Work out the finished part from the listing and answer in its coordinate system (mm). Round coordinates to 2 decimals unless told otherwise and drop trailing zeros. Write each loop counter-clockwise with the first axis right and the second up, starting at its lowest first coordinate (ties: lowest second). Pieces come first, ordered by that corner, then holes. Notation, with made-up numbers: (-37.5, -2) -> (-7.5, -2) arc R14 ccw to (-7.5, 4) -> close; hole circle Ø5 at (49, -31). An arc over 180 degrees is marked (long way). One line per item, written item: value.
```python
from build123d import *

# Parameters (mm, degrees)
SKETCH1_R                  = 1.25
BOSS_EXTRUDE1_DEPTH        = 5
BOSS_EXTRUDE2_START        = -5
BOSS_EXTRUDE2_DEPTH        = 5
F_2_0_2_DIAMETER_HOLE2_D   = 2
FILLET2_R                  = 3
F_2_8_2_8_DIAMETER_HOLE1_D = 2.8


with BuildPart() as part:
    # Sketch1 → Boss-Extrude1 (new body)
    with BuildSketch(Plane(origin=(0, 0, 0), x_dir=(1, 0, 0), z_dir=(0, 1, 0))):
        with BuildLine():
            Line((29, 74), (-29, 74))
            ThreePointArc((-29, 74), (-45.770509831, 70.041019662), (-59, 59))
            Line((-59, 59), (-59, 0))
            Line((-59, 0), (-59, -15))
            ThreePointArc((-59, -15), (-67.992720962, -23.992720962), (-76.985441925, -15))
            Line((-76.985441925, -15), (-75, 0))
            Line((-75, 0), (-75, 60))
            ThreePointArc((-75, 60), (-56.459060435, 81.837226001), (-29, 90))
            Line((-29, 90), (29, 90))
            ThreePointArc((29, 90), (56.459060435, 81.837226001), (75, 60))
            Line((75, 60), (75, 0))
            Line((75, 0), (76.985441925, -15))
            ThreePointArc((76.985441925, -15), (67.992720962, -23.992720962), (59, -15))
            Line((59, -15), (59, 0))
            Line((59, 0), (59, 59))
            ThreePointArc((59, 59), (45.770509831, 70.041019662), (29, 74))
        make_face()
        with Locations(Location((67, 5, 0), (0, 0, 270))):
            Circle(SKETCH1_R, mode=Mode.SUBTRACT)
        with Locations(Location((68.915666574, -15, 0), (0, 0, 270))):
            Circle(SKETCH1_R, mode=Mode.SUBTRACT)
        with Locations(Location((-68.915666574, -15, 0), (0, 0, 90))):
            Circle(SKETCH1_R, mode=Mode.SUBTRACT)
        with Locations(Location((-67, 5, 0), (0, 0, 90))):
            Circle(SKETCH1_R, mode=Mode.SUBTRACT)
    extrude(amount=BOSS_EXTRUDE1_DEPTH)

    # Sketch2 → Boss-Extrude2 (add)
    with BuildSketch(Plane(origin=(0, 5, 0), x_dir=(1, 0, 0), z_dir=(0, 1, 0)).offset(BOSS_EXTRUDE2_START)):
        with BuildLine():
            Line((52, 45.986664295), (59, 39.986664295))
            Line((59, 39.986664295), (59, 51.986664295))
            ThreePointArc((59, 51.986664295), (54.390227771, 50.281398562), (52, 45.986664295))
        make_face()
        with BuildLine():
            ThreePointArc((26.500025406, 74), (29.864997094, 70.489268948), (33.490587946, 73.730157398))
            ThreePointArc((33.490587946, 73.730157398), (31.249344079, 73.932478561), (29, 74))
            Line((29, 74), (26.500025406, 74))
        make_face()
        with BuildLine():
            ThreePointArc((-33.490587946, 73.730157398), (-29.864997094, 70.489268948), (-26.500025406, 74))
            Line((-26.500025406, 74), (-29, 74))
            ThreePointArc((-29, 74), (-31.249344079, 73.932478561), (-33.490587946, 73.730157398))
        make_face()
        with BuildLine():
            Line((-6.92820323, 90), (6.92820323, 90))
            ThreePointArc((6.92820323, 90), (0, 94), (-6.92820323, 90))
        make_face()
        with BuildLine():
            ThreePointArc((-52, 45.986664295), (-54.390227771, 50.281398562), (-59, 51.986664295))
            Line((-59, 51.986664295), (-59, 39.986664295))
            Line((-59, 39.986664295), (-52, 45.986664295))
        make_face()
    extrude(amount=BOSS_EXTRUDE2_DEPTH)

    # Ø2.0 (2) Diameter Hole2 (through all)
    with Locations(Plane(origin=(0, 5, 0), x_dir=(1, 0, 0), z_dir=(0, 1, 0))):
        with Locations((30, 73.986664295), (56, 47.986664295), (-30, 73.986664295), (-56, 47.986664295)):
            Hole(F_2_0_2_DIAMETER_HOLE2_D / 2)

    # Fillet2
    fillet2_edges = [part.edges().sort_by_distance(p)[0] for p in [
        (52, 2.5, -45.986664295),
        (59, 2.5, -51.986664295),
        (59, 2.5, -39.986664295),
        (59, 2.5, -59),
        (-59, 2.5, -59),
        (-75, 2.5, -60),
        (75, 2.5, -60),
        (-6.92820323, 2.5, -90),
        (6.92820323, 2.5, -90),
        (-26.500025406, 2.5, -74),
        (-33.490587946, 2.5, -73.730157398),
        (-52, 2.5, -45.986664295),
        (-59, 2.5, -39.986664295),
        (-59, 2.5, -51.986664295),
        (26.500025406, 2.5, -74),
        (33.490587946, 2.5, -73.730157398),
    ]]
    fillet(fillet2_edges, radius=FILLET2_R)

    # Ø2.8 (2.8) Diameter Hole1 (through all)
    with Locations(Plane(origin=(0, 5, 0), x_dir=(1, 0, 0), z_dir=(0, 1, 0))):
        with Locations((0, 86)):
            Hole(F_2_8_2_8_DIAMETER_HOLE1_D / 2)


solid = part.part
```
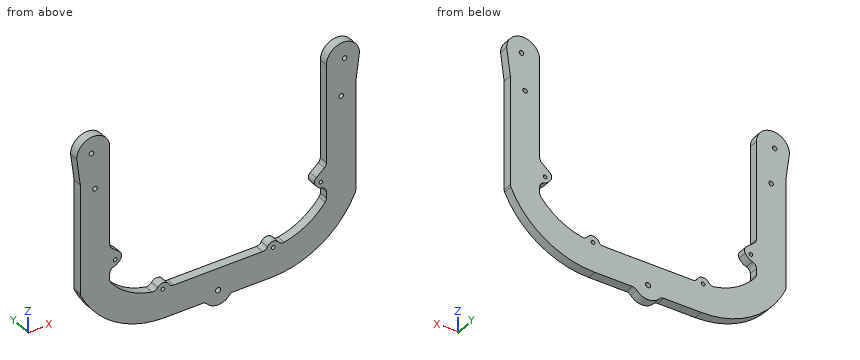
(1) Find section D-D on x = 40. Give the vertices of the cut face in (y, z).
Reported:
outline: (0, -88.78) -> (5, -88.78) -> (5, -72.35) -> (0, -72.35) -> close
(2) Flat-ended cylindrical pins translate along their axes: pin 1 Ø3 at (y, z) = (3.5, -57) entering from +X; pin 2 Ø3 at (x, y) = (-30.5, 1.5) entering from -Z; pin 3 Ø1 at (y, z) = (3.5, -61.5) entering from +X; pin 4 Ø1.5 at (x, z) = (67, -5) entering from +Y. Find the tip coordinate at first contact, or state that the pin passes through.
Reported:
pin 1: stops at x = 75
pin 2: stops at z = -90
pin 3: stops at x = 74.55
pin 4: passes through
(3) Consider probe 1 along X at (y, z) = (3.25, -32.5); probe 2 along Z at (x, y) = (30, 3); probe 3 along Z at (x, y) = (-56, 2.2). Determine where each line is inside the solid, lowest interval first.
Reported:
probe 1: x = -75 to -59, 59 to 75
probe 2: z = -89.99 to -74.99, -72.99 to -70.49
probe 3: z = -82.13 to -62.52, -51.32 to -48.99, -46.99 to -42.56
(4) Find section C-C on y = 3.75. Give the number of separate pieces and of enclosed holes in the cut face, plus the area to 3 significant figures.
Reported:
separate pieces: 1
enclosed holes: 9
area: 5,180 mm2
(5) Find section A-A on z = -22. Give the vertices of the cut face in (x, y).
Reported:
outline: (-75, 0) -> (-59, 0) -> (-59, 5) -> (-75, 5) -> close; (59, 0) -> (75, 0) -> (75, 5) -> (59, 5) -> close
(6) Find section B-B on x = 17.5. Give the vertices of the cut face in (y, z).
Reported:
outline: (0, -90) -> (5, -90) -> (5, -74) -> (0, -74) -> close
